Check sheet for the modelled part. Datum: model origin and axes. Units: mm. A direction names the side the tool comes from. Round coordinates to 2 decimals unless told otherwise and drop trailing zeros. Loops run counter-clockwise (first coordinate to the right, second up) from the corner with the lowest first, then second, coordinate; pieces in that order, holes last. Notation, with made-up numbers: (56, -27) - (61, -27) arc R31 cw to (61, 6) - close; hole circle Ø1 at (-38, 55). An arc over 180 degrees is marked (long way). Put each result on its own line as item: value. Start each with the question number.
Item 1: Gauge pin test, flat ends, axial feed: pin 1 Ø3 at (y, z) = (52.5, 2.5) entering from -X; pin 2 Ø3 at (x, z) = (-76.5, 2) entering from -Y; pin 3 Ø3 at (y, z) = (-2.5, 3.5) entering from +X. Record the tip position at first contact, or that the pin passes through.
Item 2: Draft check along X on faces 1 (the flat face through (-32.089, 53, 3)), 2 (the flat face through (-12.089, -3, 3)), 3 (the flat face through (-32.089, -3, 3)), 4 (the flat face through (-22, -5.5, 3)). Enter one of: pulls with the +X half, pulls with the -X half, needs draft (parallel to the pull), parting line crosses it, or undercut.
Item 3: Section check A-A, the plane z = 4.3. Record the cut outline in (x, y), and give its area (3 significant figures).
Item 4: Material ranges on line 1 along X through (y, z) = (-2.5, 1.3); line 2 along Y through (x, z) = (-45, 2.9), recorded low to high.
Item 5: Section check B-B, the plane x = -77. Record the cut outline in (y, z), and give its area (3 significant figures).
Item 6: Tool access check on faces 5 (the flat face through (-43, 0, 3)), 6 (the flat face through (-74.514, -3, 3)), 7 (the flat face through (-43, 50, 3)). Record the directions out of +Z, -Z, +X, -X, +Y, -Y that give a thin tool (end or side, any length) a straight path to the whole face; none if there is none.
Autodesk Inventor part; units mm, degrees
ref_plane "YZ Plane" through (0, 0, 0) normal (1, 0, 0) x (0, 1, 0)
ref_plane "XZ Plane" through (0, 0, 0) normal (0, 1, 0) x (-1, 0, 0)
ref_plane "XY Plane" through (0, 0, 0) normal (0, 0, 1) x (1, 0, 0)
sketch "Sketch1" plane through (0, 0, 0) normal (0, 0, 1) x (1, 0, 0)
  line L0 (-12.089, 0) -> (-12.089, -5.5)
  line L1 (-12.089, -5.5) -> (-32.089, -5.5)
  line L2 (-32.089, -5.5) -> (-32.089, 0)
  line L3 (-54.514, 0) -> (-54.514, -5.5)
  line L4 (-54.514, -5.5) -> (-74.514, -5.5)
  line L5 (-74.514, -5.5) -> (-74.514, 0)
  line L6 (-32.089, 0) -> (-54.514, 0)
  line L7 (-12.089, 50) -> (-12.089, 55.5)
  line L8 (-12.089, 55.5) -> (-32.089, 55.5)
  line L9 (-32.089, 55.5) -> (-32.089, 50)
  line L10 (-54.514, 50) -> (-54.514, 55.5)
  line L11 (-54.514, 55.5) -> (-74.514, 55.5)
  line L12 (-74.514, 55.5) -> (-74.514, 50)
  line L13 (-32.089, 50) -> (-54.514, 50)
  line L14 (-12.089, 0) -> (-4.089, 0)
  line L15 (-4.089, 0) -> (-4.089, 50)
  line L16 (-4.089, 50) -> (-12.089, 50)
  line L17 (-74.514, 50) -> (-82.514, 50)
  line L18 (-82.514, 50) -> (-82.514, 0)
  line L19 (-82.514, 0) -> (-74.514, 0)
  dimension "d2" = 5.5
  dimension "d3" = 20
  dimension "d4" = 5.5
  dimension "d5" = 20
  dimension "d6" = 90
  dimension "d18" = 8
  dimension "d20" = 8
extrude "Extrusion1" add sketch "Sketch1" along normal blind 5.5
properties part number "lado"
Check result:
1. pin 1: x = -74.51
1. pin 2: y = 0
1. pin 3: x = -12.09
2. face 1: undercut
2. face 2: pulls with the +X half
2. face 3: undercut
2. face 4: needs draft
3. outline: (-82.51, 0) - (-74.51, 0) - (-74.51, -5.5) - (-54.51, -5.5) - (-54.51, 0) - (-32.09, 0) - (-32.09, -5.5) - (-12.09, -5.5) - (-12.09, 0) - (-4.09, 0) - (-4.09, 50) - (-12.09, 50) - (-12.09, 55.5) - (-32.09, 55.5) - (-32.09, 50) - (-54.51, 50) - (-54.51, 55.5) - (-74.51, 55.5) - (-74.51, 50) - (-82.51, 50) - close
3. area: 4,360 mm²
4. line 1: -74.51 to -54.51, -32.09 to -12.09
4. line 2: 0 to 50
5. outline: (0, 0) - (50, 0) - (50, 5.5) - (0, 5.5) - close
5. area: 275 mm²
6. face 5: +Z, -Z, -Y
6. face 6: +Z, -Z, -X, -Y
6. face 7: +Z, -Z, +Y
